Could you check a few things on this model? Use its own coordinates, in mm. Round coordinates to 2 decimals unless told otherwise and drop trailing zeros. Order: outer loops, then holes, each group sorted by start corner. A loop starts at its lowest first (then second) coordinate and runs counter-clockwise, first axis right, second up. Notation, with made-up numbers: (36, -34.75) - (73, -34.75) arc R31 cw to (73, -8.75) - close; hole circle Ø4 at (-32, 41). An arc over 180 degrees is marked (long way). Use one line per item in the form item = value.
from build123d import *

# Parameters (mm, degrees)
SKETCH_1_W                   = 90
SKETCH_1_H                   = 90
EXTRUDE_1_DEPTH              = 5
FILLET_1_R                   = 10
HOLE_WIZARD_M6_1_D           = 5
HOLE_WIZARD_M6_1_DEPTH       = 17
HOLE_WIZARD_M6_1_CSINK_D     = 6.05
HOLE_WIZARD_M6_1_CSINK_ANGLE = 90
HOLE_WIZARD_M6_1_TIP         = 1.502151548
SKETCH_4_R                   = 40
CUT_EXTRUDE_1_DEPTH          = 2


with BuildPart() as part:
    # 草图1 → 凸台-拉伸1 (new body)
    with BuildSketch(Plane.XY):
        Rectangle(SKETCH_1_W, SKETCH_1_H)
    extrude(amount=EXTRUDE_1_DEPTH)

    # 圆角1
    fillet_1_edges = [part.edges().sort_by_distance(p)[0] for p in [
        (45, -45, 2.5),
        (-45, -45, 2.5),
        (-45, 45, 2.5),
        (45, 45, 2.5),
    ]]
    fillet(fillet_1_edges, radius=FILLET_1_R)

    # M6 螺纹孔1
    with Locations(Plane.XY.offset(5)):
        with Locations((35.355339059, -35.355339059), (-35.355339059, 35.355339059), (35.355339059, 35.355339059), (-35.355339059, -35.355339059)):
            CounterSinkHole(HOLE_WIZARD_M6_1_D / 2, HOLE_WIZARD_M6_1_CSINK_D / 2, depth=HOLE_WIZARD_M6_1_DEPTH, counter_sink_angle=HOLE_WIZARD_M6_1_CSINK_ANGLE)
            with Locations((0, 0, -(HOLE_WIZARD_M6_1_DEPTH + HOLE_WIZARD_M6_1_TIP / 2))):  # 118° drill point
                Cone(0, HOLE_WIZARD_M6_1_D / 2, HOLE_WIZARD_M6_1_TIP, mode=Mode.SUBTRACT)

    # 草图4 → 切除-拉伸1 (cut)
    with BuildSketch(Plane.XY.offset(5)):
        Circle(SKETCH_4_R)
    extrude(amount=-CUT_EXTRUDE_1_DEPTH, mode=Mode.SUBTRACT)


solid = part.part
Item 1: Imagine slicing it at B-B on z = 0.75. Please give me the cut outline in (x, y), plus the area to 3 significant figures.
Found:
outline = (-45, -35) arc R10 ccw to (-35, -45) - (35, -45) arc R10 ccw to (45, -35) - (45, 35) arc R10 ccw to (35, 45) - (-35, 45) arc R10 ccw to (-45, 35) - close; hole circle Ø5 at (-35.36, -35.36); hole circle Ø5 at (-35.36, 35.36); hole circle Ø5 at (35.36, -35.36); hole circle Ø5 at (35.36, 35.36)
area = 7,940 mm2
Item 2: Will this pin go through, and if not, where does the flat tip stop? P1, Ø4, axis at x = 9, y = 5.5, coming from the +Z side.
Found:
P1 = 3
Item 3: Imagine slicing it at A-A on x = 0. Please give me the cut outline in (y, z), plus the area to 3 significant figures.
Found:
outline = (-45, 0) - (45, 0) - (45, 5) - (40, 5) - (40, 3) - (-40, 3) - (-40, 5) - (-45, 5) - close
area = 290 mm2
Item 4: I need wall thicknesses on L1, parallel to Y at x = -35, z = 2.2; L2, parallel to Z at x = -23, y = -6.5; L3, parallel to X at y = 37, z = 1.55. Which ranges of each line are inside material? Lowest first, please.
Found:
L1 = -45 to -37.83, -32.88 to 32.88, 37.83 to 45
L2 = 0 to 3
L3 = -44.8 to -37.24, -33.47 to 33.47, 37.24 to 44.8
